from build123d import *

# Parameters (mm, degrees)
BOSS_EXTRUDE1_DEPTH = 10
FILLET1_R           = 10
FILLET2_R           = 5
SKETCH2_W           = 35
SKETCH2_H           = 15.070963555
CUT_EXTRUDE1_DEPTH  = 4


with BuildPart() as part:
    # Sketch1 → Boss-Extrude1 (new body)
    with BuildSketch(Plane.XY):
        Polygon((-7.5, 467.320715151), (-7.5, 500.037974444), (-12.25, 508.842566049), (-12.25, 526.07117063), (-6.25, 526.07117063), (-6.25, 511.000207075), (16.75, 511.000207075), (16.75, 526.07117063), (22.75, 526.07117063), (22.75, 508.842566049), (7.5, 500.037974444), (7.5, 467.320715151), align=None)
    extrude(amount=BOSS_EXTRUDE1_DEPTH)

    # Fillet1
    fillet1_edges = [part.edges().sort_by_distance(p)[0] for p in [
        (7.5, 500.037974444, 5),
        (-7.5, 500.037974444, 5),
    ]]
    fillet(fillet1_edges, radius=FILLET1_R)

    # Fillet2
    fillet2_edges = [part.edges().sort_by_distance(p)[0] for p in [
        (22.75, 508.842566049, 5),
        (-12.25, 508.842566049, 5),
    ]]
    fillet(fillet2_edges, radius=FILLET2_R)

    # Sketch2 → Cut-Extrude1 (cut)
    with BuildSketch(Plane.XY.offset(10)):
        with Locations((5.25, 518.535688853)):
            Rectangle(SKETCH2_W, SKETCH2_H)
    extrude(amount=-CUT_EXTRUDE1_DEPTH, mode=Mode.SUBTRACT)


solid = part.part
Could you check a few things on this model? Use its own coordinates, in mm. A direction names the side the tool comes from. Give positions to 0.01 mm unless a question says otherwise; leave off trailing zeros. Write each loop counter-clockwise with the first axis right and the second up, starting at its lowest first coordinate (ties: lowest second). Pieces come first, ordered by that corner, then holes. Notation, with made-up numbers: (4, 20) - (21, 20) arc R26 cw to (21, 43) - close; hole circle Ø4 at (13, 17). An arc over 180 degrees is marked (long way). Use CSV: the item, a comma, the result in double quotes. Start each with the question number.
Item 1: I'm going to push flat-ended pins straight in: pin 1 (5 mm diameter, centred on y = 488, z = 7, fed in from -X); pin 2 (3 mm diameter, centred on x = 18.5, z = 6.5, fed in from -Y); pin 3 (1 mm diameter, centred on x = 18, z = 8, fed in from +Y). Where does each tip first touch, or does it pass through?
Item 2: I want a section at A-A, the plane y = 514.5. Please give me the cut outline in (x, z).
Item 3: I want a section at C-C, the plane z = 2.5. Please give me the cut outline in (x, y), then the cut area to 3 significant figures.
Item 4: If we mould it in two halves opening along X, with no side actions, what happens to faces 4 (the face through (-6.25, 519, 3)), 5 (the face through (22.75, 519, 3)), 6 (the face through (-12.25, 518, 3))? For each: pulls with the +X half, pulls with the -X half, needs draft (parallel to the pull), parting line crosses it, or undercut.
Item 5: I want a section at B-B, the plane z = 6.75. Please give me the cut outline in (x, y), then the cut area to 3 significant figures.
Item 6: I want a section at D-D, the plane x = 8.5. Please give me the cut outline in (y, z).
Item 7: If I drill on line 1 along X through (y, z) = (521.5, 2.75); line 2 along X through (y, z) = (487, 3.5); line 3 along Y through (x, z) = (-0.5, 5.5), over which ranges is the centre line in solid material (lowest first)?
Item 8: For faces 1 (the face through (-7.5, 482, 5)), 2 (the face through (-9, 519, 6)), 3 (the face through (7.5, 481, 5)), which set-ups out of +Z, -Z, +X, -X, +Y, -Y let a thin tool reach every point of the face, with its end or its side?
Findings:
1,pin 1,"stops at x = -7.5"
1,pin 2,"stops at y = 505.52"
1,pin 3,"stops at y = 511"
2,outline,"(-12.25, 0) - (-6.25, 0) - (-6.25, 6) - (-12.25, 6) - close; (16.75, 0) - (22.75, 0) - (22.75, 6) - (16.75, 6) - close"
3,outline,"(-12.25, 510.11) arc R5 ccw to (-11.65, 507.73) - (-8.7, 502.26) arc R10 cw to (-7.5, 497.51) - (-7.5, 467.32) - (7.5, 467.32) - (7.5, 494.26) arc R10 cw to (12.5, 502.92) - (20.25, 507.4) arc R5 ccw to (22.75, 511.73) - (22.75, 526.07) - (16.75, 526.07) - (16.75, 511) - (-6.25, 511) - (-6.25, 526.07) - (-12.25, 526.07) - close"
3,area,"972 mm2"
4,face 4,"undercut"
4,face 5,"pulls with the +X half"
4,face 6,"pulls with the -X half"
5,outline,"(-12.25, 510.11) arc R5 ccw to (-11.65, 507.73) - (-8.7, 502.26) arc R10 cw to (-7.5, 497.51) - (-7.5, 467.32) - (7.5, 467.32) - (7.5, 494.26) arc R10 cw to (12.5, 502.92) - (20.25, 507.4) arc R5 ccw to (22.7, 511) - (-12.25, 511) - close"
5,area,"791 mm2"
6,outline,"(498.62, 0) - (511, 0) - (511, 10) - (498.62, 10) - close"
7,line 1,"x = -12.25 to -6.25, 16.75 to 22.75"
7,line 2,"x = -7.5 to 7.5"
7,line 3,"y = 467.32 to 511"
8,face 1,"+Z, -Z, -X, -Y"
8,face 2,"+Z, +X, -X, +Y"
8,face 3,"+Z, -Z, +X, -Y"
